Could you check a few things on this model? Use its own coordinates, in mm. Face numbers are marked on the shaded views. A direction names the side the tool comes from. Coordinates: 2 decimals unless noted, no trailing zeros. Order: outer loops, then holes, each group sorted by start corner. A loop starts at its lowest first (then second) coordinate and runs counter-clockwise, first axis right, second up. Notation, with made-up numbers: (78.25, 66) -> (116.25, 66) arc R26 ccw to (116.25, 99) -> close; hole circle Ø7 at (-8, 10). An arc over 180 degrees is marked (long way). Return JSON: item names as keys, results as strings. Group by question number.
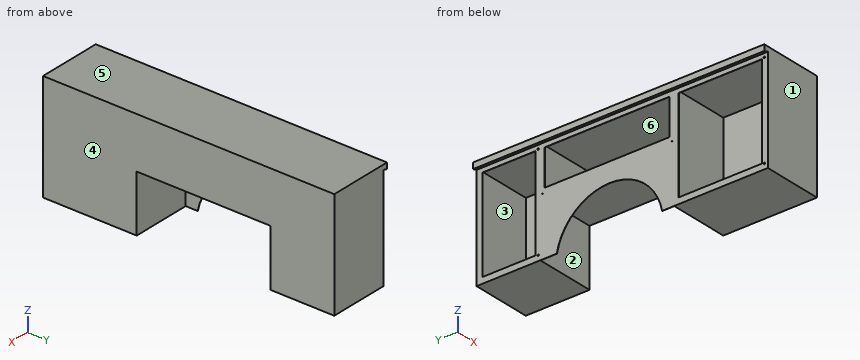
from build123d import *

# Parameters (mm, degrees)
F0_W      = 508
F0_H      = 914.4
F1_DEPTH  = 2470.15
F2_W      = 450.85
F2_H      = 787.4
F2_W_2    = 1060.45
F2_H_2    = 304.8
F2_W_3    = 704.85
F3_DEPTH  = 505.8918
F4_W      = 503.7836
F4_H      = 704.85
F5_DEPTH  = 48.6918
F6_W      = 503.7836
F6_H      = 704.85
F7_DEPTH  = 48.6918
F8_W      = 503.7836
F8_H      = 884.7836
F9_DEPTH  = 37.0459
F10_W     = 503.7836
F10_H     = 884.7836
F11_DEPTH = 48.6918
F12_W     = 503.7836
F12_H     = 1060.45
F13_DEPTH = 48.6918
F14_W     = 503.7836
F14_H     = 1060.45
F15_DEPTH = 48.6918
F16_W     = 503.7836
F16_H     = 402.1836
F17_DEPTH = 37.0459
F18_W     = 503.7836
F18_H     = 402.1836
F19_DEPTH = 37.0459
F20_W     = 503.7836
F20_H     = 450.85
F21_DEPTH = 48.6918
F22_W     = 503.7836
F22_H     = 450.85
F23_DEPTH = 48.6918
F24_W     = 503.7836
F24_H     = 884.7836
F25_DEPTH = 37.0459
F26_W     = 503.7836
F26_H     = 884.7836
F27_DEPTH = 48.6918
F28_W     = 505.8918
F28_H     = 1134.5418
F29_DEPTH = 482.6
F31_DEPTH = 508.001
F33_DEPTH = 2470.15
F34_R     = 0.508
F35_R     = 3.175
F36_DEPTH = 2.1082
F37_R     = 6.35
F38_DEPTH = 2.1082
F39_R     = 6.35
F40_DEPTH = 2.1082


# Not quite as in the source:
# - a feature names something its author has since deleted; it is built from what else it names


with BuildPart() as f1:
    # F0 (on Front) → F1 (new body)
    with BuildSketch(Plane.XZ):
        Rectangle(F0_W, F0_H)
    extrude(amount=-F1_DEPTH)

    # F2 (on face) → F3 (cut)
    with BuildSketch(Plane(origin=(-254, 0, 0), x_dir=(0, -1, 0), z_dir=(-1, 0, 0))):
        with Locations((-2193.925, -12.7)):
            Rectangle(F2_W, F2_H)
        with Locations((-1362.075, 228.6)):
            Rectangle(F2_W_2, F2_H_2)
        with Locations((-403.225, -12.7)):
            Rectangle(F2_W_3, F2_H)
    extrude(amount=-F3_DEPTH, mode=Mode.SUBTRACT)

    # F4 (on face) → F5 (cut)
    with BuildSketch(Plane.XY.offset(-406.4)):
        with Locations((0, 403.225)):
            Rectangle(F4_W, F4_H)
    extrude(amount=-F5_DEPTH, mode=Mode.SUBTRACT)

    # F6 (on face) → F7 (cut)
    with BuildSketch(Plane(origin=(0, 0, 381), x_dir=(1, 0, 0), z_dir=(0, 0, -1))):
        with Locations((0, -403.225)):
            Rectangle(F6_W, F6_H)
    extrude(amount=-F7_DEPTH, mode=Mode.SUBTRACT)

    # F8 (on face) → F9 (cut)
    with BuildSketch(Plane.XZ.offset(-755.65)):
        with Locations((0, -12.7)):
            Rectangle(F8_W, F8_H)
    extrude(amount=-F9_DEPTH, mode=Mode.SUBTRACT)

    # F10 (on face) → F11 (cut)
    with BuildSketch(Plane(origin=(0, 50.8, 0), x_dir=(-1, 0, 0), z_dir=(0, 1, 0))):
        with Locations((0, -12.7)):
            Rectangle(F10_W, F10_H)
    extrude(amount=-F11_DEPTH, mode=Mode.SUBTRACT)

    # F12 (on face) → F13 (cut)
    with BuildSketch(Plane.XY.offset(76.2)):
        with Locations((0, 1362.075)):
            Rectangle(F12_W, F12_H)
    extrude(amount=-F13_DEPTH, mode=Mode.SUBTRACT)

    # F14 (on face) → F15 (cut)
    with BuildSketch(Plane(origin=(0, 0, 381), x_dir=(1, 0, 0), z_dir=(0, 0, -1))):
        with Locations((0, -1362.075)):
            Rectangle(F14_W, F14_H)
    extrude(amount=-F15_DEPTH, mode=Mode.SUBTRACT)

    # F16 (on face) → F17 (cut)
    with BuildSketch(Plane(origin=(0, 831.85, 0), x_dir=(-1, 0, 0), z_dir=(0, 1, 0))):
        with Locations((0, 228.6)):
            Rectangle(F16_W, F16_H)
    extrude(amount=-F17_DEPTH, mode=Mode.SUBTRACT)

    # F18 (on face) → F19 (cut)
    with BuildSketch(Plane.XZ.offset(-1892.3)):
        with Locations((0, 228.6)):
            Rectangle(F18_W, F18_H)
    extrude(amount=-F19_DEPTH, mode=Mode.SUBTRACT)

    # F20 (on face) → F21 (cut)
    with BuildSketch(Plane.XY.offset(-406.4)):
        with Locations((0, 2193.925)):
            Rectangle(F20_W, F20_H)
    extrude(amount=-F21_DEPTH, mode=Mode.SUBTRACT)

    # F22 (on face) → F23 (cut)
    with BuildSketch(Plane(origin=(0, 0, 381), x_dir=(1, 0, 0), z_dir=(0, 0, -1))):
        with Locations((0, -2193.925)):
            Rectangle(F22_W, F22_H)
    extrude(amount=-F23_DEPTH, mode=Mode.SUBTRACT)

    # F24 (on face) → F25 (cut)
    with BuildSketch(Plane(origin=(0, 1968.5, 0), x_dir=(-1, 0, 0), z_dir=(0, 1, 0))):
        with Locations((0, -12.7)):
            Rectangle(F24_W, F24_H)
    extrude(amount=-F25_DEPTH, mode=Mode.SUBTRACT)

    # F26 (on face) → F27 (cut)
    with BuildSketch(Plane.XZ.offset(-2419.35)):
        with Locations((0, -12.7)):
            Rectangle(F26_W, F26_H)
    extrude(amount=-F27_DEPTH, mode=Mode.SUBTRACT)

    # F28 (on face) → F29 (cut)
    with BuildSketch(Plane(origin=(0, 0, -457.2), x_dir=(1, 0, 0), z_dir=(0, 0, -1))):
        with Locations((1.0541, -1362.075)):
            Rectangle(F28_W, F28_H)
    extrude(amount=-F29_DEPTH, mode=Mode.SUBTRACT)

    # F30 (on face) → F31 (cut, through all)
    with BuildSketch(Plane(origin=(-254, 0, 0), x_dir=(0, -1, 0), z_dir=(-1, 0, 0))):
        with BuildLine():
            Line((-1789.6459, -457.2), (-896.4041, -457.2))
            ThreePointArc((-896.4041, -457.2), (-1343.025, -86.7918), (-1789.6459, -457.2))
        make_face()
    extrude(amount=-F31_DEPTH, mode=Mode.SUBTRACT)

    # F32 (on face) → F33 (join, through all)
    with BuildSketch(Plane.XZ):
        Polygon((-290.5981389248, 459.3082), (-290.5981389248, 408.5082), (-254, 419.1), (-254, 457.2), (254, 457.2), (254, 459.3082), align=None)
    extrude(amount=-F33_DEPTH)

    # F34
    f34_edges = [f1.edges().sort_by_distance(p)[0] for p in [
        (-290.598139, 1235.075, 408.5082),
    ]]
    fillet(f34_edges, radius=F34_R)

    # F35 (on face) → F36 (cut, through all)
    with BuildSketch(Plane(origin=(-254, 0, 0), x_dir=(0, -1, 0), z_dir=(-1, 0, 0))):
        with Locations((-1911.35, 38.1)):
            Circle(F35_R)
        with Locations((-812.8, 38.1)):
            Circle(F35_R)
    extrude(amount=-F36_DEPTH, mode=Mode.SUBTRACT)

    # F37 (on face) → F38 (cut, through all)
    with BuildSketch(Plane(origin=(-254, 0, 0), x_dir=(0, -1, 0), z_dir=(-1, 0, 0))):
        with Locations((-29.21, 387.35)):
            Circle(F37_R)
        with Locations((-29.21, -412.75)):
            Circle(F37_R)
    extrude(amount=-F38_DEPTH, mode=Mode.SUBTRACT)

    # F39 (on face) → F40 (cut, through all)
    with BuildSketch(Plane(origin=(-254, 0, 0), x_dir=(0, -1, 0), z_dir=(-1, 0, 0))):
        with Locations((-1946.91, 387.35)):
            Circle(F39_R)
        with Locations((-1946.91, -412.75)):
            Circle(F39_R)
    extrude(amount=-F40_DEPTH, mode=Mode.SUBTRACT)


solid = f1.part
Q1. I want a section at D-D on z = 239.5. Please give me the cut outline in (x, y), and give its area (3 significant figures).
Q2. I need wall thicknesses on line 1 along Y through (x, z) = (-68.5, 139); line 2 along Z through (x, y) = (-253, 29); line 3 along Y through (x, z) = (-252, 387). Which ranges of each line are inside material? Lowest first, please. Write a range as from..to.
Q3. I want a section at A-A on x = 3. Please give me the cut outline in (y, z), and give its area (3 significant figures).
Q4. I'm going to push flat-ended pins straight in: pin 1 Ø10 at (x, z) = (196, -200) entering from -Y; pin 2 Ø4 at (y, z) = (1609, -76) entering from -X. Where does each tip first touch, or does it pass through?
Q5. I want a section at B-B on z = -183.5. Please give me the cut outline in (x, y), and give its area (3 significant figures).
Q6. On a 3-axis mill with a long thin cutter (end or side, diameter ignored), from which of +Z, -Z, +X, -X, +Y, -Y can I reach the whole of each face in a straight line? I mean the marked faces 1, 2 and 3. Say none if no direction works.
Q7. I want a section at C-C on y = 614.5. Please give me the cut outline in (x, z), and give its area (3 significant figures).
Q8. We'd pull the mould along X, two halves only. Please class the marked faces 4, 5 and 6: pulls with the +X half, pulls with the -X half, needs draft (parallel to the pull), parting line crosses it, or undercut.
Response values:
{
 "1": {"outline": "(-254, 0) -> (254, 0) -> (254, 2470.15) -> (-254, 2470.15) -> (-254, 2419.35) -> (-251.89, 2419.35) -> (-251.89, 2468.04) -> (251.89, 2468.04) -> (251.89, 1931.45) -> (-251.89, 1931.45) -> (-251.89, 1968.5) -> (-254, 1968.5) -> (-254, 1892.3) -> (-251.89, 1892.3) -> (-251.89, 1929.35) -> (251.89, 1929.35) -> (251.89, 794.8) -> (-251.89, 794.8) -> (-251.89, 831.85) -> (-254, 831.85) -> (-254, 755.65) -> (-251.89, 755.65) -> (-251.89, 792.7) -> (251.89, 792.7) -> (251.89, 2.11) -> (-251.89, 2.11) -> (-251.89, 50.8) -> (-254, 50.8) -> close", "area": "9,990 mm²"},
 "2": {"line 1": "y = 0..2.11, 792.7..794.8, 1929.35..1931.45, 2468.04..2470.15", "line 2": "z = -457.2..-419.1, -406.4..381, 393.7..459.31", "line 3": "y = 0..22.87, 35.55..1940.57, 1953.25..2470.15"},
 "3": {"outline": "(0, -457.2) -> (794.8, -457.2) -> (794.8, 25.4) -> (1929.35, 25.4) -> (1929.35, -457.2) -> (2470.15, -457.2) -> (2470.15, 459.31) -> (0, 459.31) -> close; hole (2.11, -455.09) -> (792.7, -455.09) -> (792.7, 429.69) -> (2.11, 429.69) -> close; hole (794.8, 27.51) -> (1929.35, 27.51) -> (1929.35, 429.69) -> (794.8, 429.69) -> close; hole (1931.45, -455.09) -> (2468.04, -455.09) -> (2468.04, 429.69) -> (1931.45, 429.69) -> close", "area": "85,800 mm²"},
 "4": {"pin 1": "stops at y = 0", "pin 2": "stops at x = -254"},
 "5": {"outline": "(-254, 0) -> (254, 0) -> (254, 794.8) -> (-251.89, 794.8) -> (-251.89, 1062.76) -> (-254, 1062.76) -> (-254, 755.65) -> (-251.89, 755.65) -> (-251.89, 792.7) -> (251.89, 792.7) -> (251.89, 2.11) -> (-251.89, 2.11) -> (-251.89, 50.8) -> (-254, 50.8) -> close; (-254, 1623.29) -> (-251.89, 1623.29) -> (-251.89, 1929.35) -> (254, 1929.35) -> (254, 2470.15) -> (-254, 2470.15) -> (-254, 2419.35) -> (-251.89, 2419.35) -> (-251.89, 2468.04) -> (251.89, 2468.04) -> (251.89, 1931.45) -> (-251.89, 1931.45) -> (-251.89, 1968.5) -> (-254, 1968.5) -> close", "area": "8,650 mm²"},
 "6": {"face 1": "+Z, -Z, +X, -X, -Y", "face 2": "-Z, +X", "face 3": "none"},
 "7": {"outline": "(-290.6, 409.18) arc R0.51 ccw to (-289.95, 408.7) -> (-254, 419.1) -> (-254, 381) -> (-251.89, 381) -> (-251.89, 429.69) -> (251.89, 429.69) -> (251.89, -455.09) -> (-251.89, -455.09) -> (-251.89, -406.4) -> (-254, -406.4) -> (-254, -457.2) -> (254, -457.2) -> (254, 459.31) -> (-290.6, 459.31) -> close", "area": "19,900 mm²"},
 "8": {"face 4": "pulls with the +X half", "face 5": "needs draft", "face 6": "undercut"}
}
